Here's the drawing with two shaded views (mm, measured from the low corner). I have some questions. A direction names the side the tool comes from. Coordinates: 2 decimals unless noted, no trailing zeros. Write each loop counter-clockwise with the first axis right and the second up, starting at its lowest first coordinate (ties: lowest second). Pieces come first, ordered by that corner, then holes.
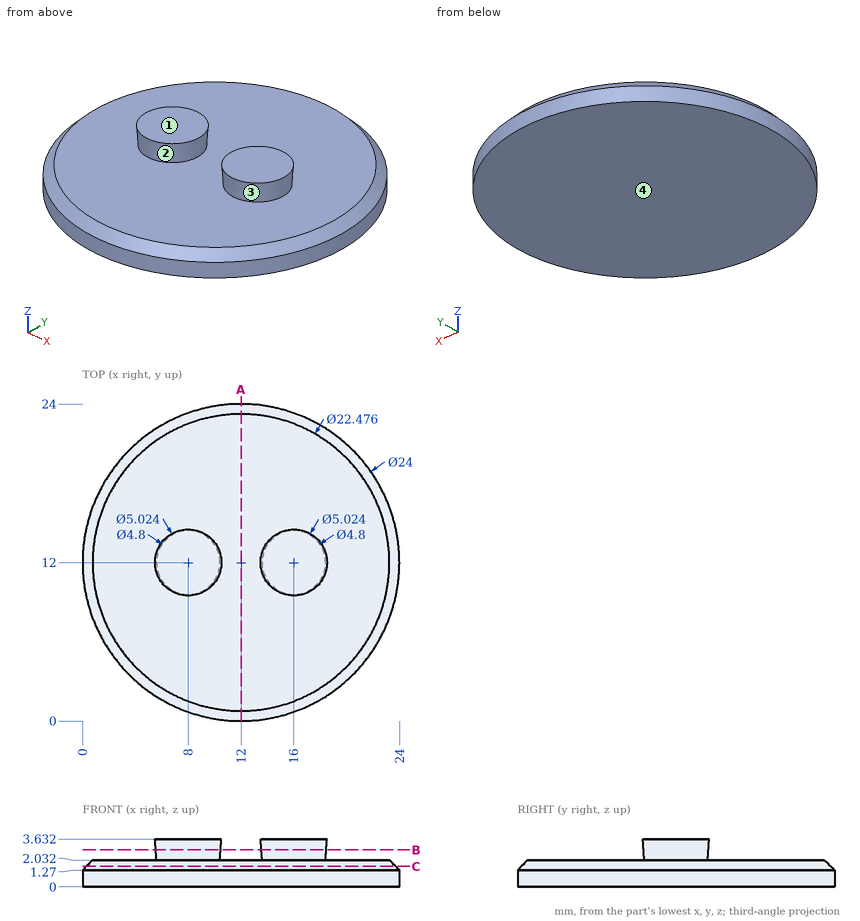
1. I want a section at B-B on z = 2.8. Please give me the cut outline in (x, y), plus the area to 3 significant figures.
Verdict:
outline: circle Ø4.91 at (8, 12); circle Ø4.91 at (16, 12)
area: 37.8 mm2
2. I want a section at C-C on z = 1.55. Please give me the cut outline in (x, y).
Verdict:
outline: circle Ø23.44 at (12, 12)
3. For pin 1 (3 mm diameter, centred on x = 5.5, y = 18.5, fed in from +Z); pin 2 (1.5 mm diameter, centred on x = 6.5, z = 3, fed in from -Y), each with a flat end and sliding along its axis, tell me the tip position at first contact or that it passes through.
Verdict:
pin 1: stops at z = 2.03
pin 2: stops at y = 9.64
4. On a 3-axis mill with a long thin cutter (end or side, diameter ignored), from which of +Z, -Z, +X, -X, +Y, -Y can I reach the whole of each face in a straight line? I mean the marked faces 3 and 4. Say none if no direction works.
Verdict:
face 3: none
face 4: -Z, +X, -X, +Y, -Y
5. If we mould it in two halves opening along X, with no side actions, what happens to the marked faces 1 and 2? For each: pulls with the +X half, pulls with the -X half, needs draft (parallel to the pull), parting line crosses it, or undercut.
Verdict:
face 1: needs draft
face 2: undercut
6. I want a section at A-A on x = 12. Please give me the cut outline in (y, z), plus the area to 3 significant figures.
Verdict:
outline: (0, 0) - (24, 0) - (24, 1.27) - (23.24, 2.03) - (0.76, 2.03) - (0, 1.27) - close
area: 48.2 mm2
7. Please list where these lines run through material, in increasing order: line 1 along Z through (x, y) = (20, 5.75); line 2 along Y through (x, z) = (4.75, 1.9); line 3 along X through (y, z) = (14.5, 1.5).
Verdict:
line 1: z = 0 to 2.03
line 2: y = 3.24 to 20.76
line 3: x = 0.5 to 23.5
